from build123d import *

# Parameters (mm, degrees)
SKETCH1_R           = 3.175
BOSS_EXTRUDE1_DEPTH = 12
SKETCH2_R           = 3.175
BOSS_EXTRUDE2_DEPTH = 22
CUT_EXTRUDE1_DEPTH  = 5
CUT_EXTRUDE2_DEPTH  = 30


with BuildPart() as part:
    # Sketch1 → Boss-Extrude1 (new body)
    with BuildSketch(Plane.XY):
        with BuildLine():
            Line((0, 9), (150, 9))
            ThreePointArc((150, 9), (159, 0), (150, -9))
            Line((150, -9), (0, -9))
            ThreePointArc((0, -9), (-9, 0), (0, 9))
        make_face()
        Circle(SKETCH1_R, mode=Mode.SUBTRACT)
        with Locations((150, 0)):
            Circle(SKETCH1_R, mode=Mode.SUBTRACT)
    extrude(amount=BOSS_EXTRUDE1_DEPTH)

    # Sketch2 → Boss-Extrude2 (add)
    with BuildSketch(Plane(origin=(0, 0, 0), x_dir=(-1, 0, 0), z_dir=(0, 0, -1))):
        with BuildLine():
            Line((-150, 9), (-130, 9))
            ThreePointArc((-130, 9), (-121, 0), (-130, -9))
            Line((-130, -9), (-150, -9))
            ThreePointArc((-150, -9), (-159, 0), (-150, 9))
        make_face()
        with Locations((-150, 0)):
            Circle(SKETCH2_R, mode=Mode.SUBTRACT)
    extrude(amount=BOSS_EXTRUDE2_DEPTH)

    # Sketch3 → Cut-Extrude1 (cut)
    with BuildSketch(Plane.XY.offset(12)):
        with BuildLine():
            Line((18, 6.5), (113, 6.5))
            ThreePointArc((113, 6.5), (119.5, 0), (113, -6.5))
            Line((113, -6.5), (18, -6.5))
            ThreePointArc((18, -6.5), (11.5, 0), (18, 6.5))
        make_face()
    cut_extrude1 = extrude(amount=-CUT_EXTRUDE1_DEPTH, mode=Mode.SUBTRACT)

    # Mirror1: Cut-Extrude1 across plane
    add(cut_extrude1.mirror(Plane.XY.offset(6)), mode=Mode.SUBTRACT)

    # Sketch4 → Cut-Extrude2 (cut)
    with BuildSketch(Plane(origin=(0, 0, -22), x_dir=(-1, 0, 0), z_dir=(0, 0, -1))):
        with BuildLine():
            Line((-130, 6), (-138, 6))
            ThreePointArc((-138, 6), (-144, 0), (-138, -6))
            Line((-138, -6), (-130, -6))
            ThreePointArc((-130, -6), (-124, 0), (-130, 6))
        make_face()
    extrude(amount=-CUT_EXTRUDE2_DEPTH, mode=Mode.SUBTRACT)


solid = part.part
The model under review builds one solid part; all positions refer to its coordinate system, in mm. A direction names the side the tool comes from. Round coordinates to 2 decimals unless told otherwise and drop trailing zeros. Loops run counter-clockwise (first coordinate to the right, second up) from the corner with the lowest first, then second, coordinate; pieces in that order, holes last. Notation, with made-up numbers: (57, 53.25) -> (81, 53.25) arc R9 ccw to (81, 70.25) -> close; hole circle Ø7 at (-34.5, 20.5). An arc over 180 degrees is marked (long way). Return JSON: item names as keys, results as strings.
(1) Add section A-A on y = 0. Write out the cut boundary in (x, z) (3 decimals), plus the area to 3 significant figures.
Solved:
{"outline": "(-9, 0) -> (-3.175, 0) -> (-3.175, 12) -> (-9, 12) -> close; (3.175, 0) -> (11.5, 0) -> (11.5, 5) -> (119.5, 5) -> (119.5, 0) -> (121, 0) -> (121, -22) -> (124, -22) -> (124, 8) -> (144, 8) -> (144, -22) -> (146.825, -22) -> (146.825, 12) -> (119.5, 12) -> (119.5, 7) -> (11.5, 7) -> (11.5, 12) -> (3.175, 12) -> close; (153.175, -22) -> (159, -22) -> (159, 12) -> (153.175, 12) -> close", "area": "880 mm2"}
(2) For pin 1 (6.5 mm diameter, centred on x = 74, y = -0.5, fed in from +Z); pin 2 (1 mm diameter, centred on y = 2, z = -4, fed in from -X); pin 3 (2 mm diameter, centred on y = 1, z = -7.5, fed in from -X), all flat-tipped, find the tip position at first contact; note any pin that passes through.
Solved:
{"pin 1": "z = 7", "pin 2": "x = 121.13", "pin 3": "x = 121"}
(3) For line 1 (X direction, y = 0, z = -5) (3 decimals); line 2 (Y direction, x = 150, z = -5) (3 decimals); line 3 (Z direction, x = 114, y = -7.25), list the stretches that pass through material, from the lowest coordinate up.
Solved:
{"line 1": "121 to 124, 144 to 146.825, 153.175 to 159", "line 2": "-9 to -3.175, 3.175 to 9", "line 3": "0 to 12"}
(4) For faces 4 (the flat face through (66, 0, 7)), 5 (the flat face through (66, 0, 5)), 6 (the flat face through (91, -9, 3)), list the 3-axis set-ups (+Z, -Z, +X, -X, +Y, -Y) from which the entire face can be reached by the end or side of a thin tool; tool diameter is ignored.
Solved:
{"face 4": "+Z", "face 5": "-Z", "face 6": "+Z, -Z, +X, -X, -Y"}
(5) Add section B-B on x = 92.5. Write out the cut boundary in (y, z), plus the area to 3 significant figures.
Solved:
{"outline": "(-9, 0) -> (-6.5, 0) -> (-6.5, 5) -> (6.5, 5) -> (6.5, 0) -> (9, 0) -> (9, 12) -> (6.5, 12) -> (6.5, 7) -> (-6.5, 7) -> (-6.5, 12) -> (-9, 12) -> close", "area": "86.0 mm2"}
(6) The part is to be moulded in two halves that separate along X. For faces 1 (the flat face through (144, 2, -22)), 2 (the flat face through (134, 0, 8)), 3 (the cylindrical face through (-9, 0, 6)), say which applies: released by +X, released by -X, zero draft, split by the parting line, or undercut.
Solved:
{"face 1": "zero draft", "face 2": "undercut", "face 3": "released by -X"}
